Part model, mm, in its own coordinate system. Give positions to 0.01 mm unless a question says otherwise; leave off trailing zeros. Loops run counter-clockwise (first coordinate to the right, second up) from the corner with the lowest first, then second, coordinate; pieces in that order, holes last. Notation, with made-up numbers: M 26,22.25 L 51,22.25 A21 ccw 51,27.25 Z; hole C -35.75,17 d11. An arc over 180 degrees is marked long. Answer in a Markdown table with one row per item.
from build123d import *

# Parameters (mm, degrees)
F1_DEPTH = 3
F2_W     = 55
F2_H     = 3
F3_DEPTH = 60
F5_DEPTH = 3.001
F6_R     = 1.5
F7_DEPTH = 25


with BuildPart() as f1:
    # F0 (on Front) → F1 (new body)
    with BuildSketch(Plane.XZ):
        Polygon((9.642301, -72.468617), (5.525627, -158.370032), (60.462578, -161.002788), (64.579252, -75.101374), (66.01405, -46.877436), (66.01405, -14.442657), (58.229018, -14.069573), (56.766827, -18.181978), (54.847706, -20.834833), (52.745808, -22.111611), (27.019382, -20.834833), (25.082963, -19.47934), (23.824289, -16.671533), (22.565616, -12.120947), (14.142194, -11.443201), (11.49178, -42.476468), align=None)
        Polygon((13.504524, -137.123708), (10.295481, -136.96992), (11.250439, -117.043101), (14.459482, -117.196889), align=None, mode=Mode.SUBTRACT)
        Polygon((59.128299, -119.856104), (58.201853, -139.597923), (54.832633, -139.664747), (55.769612, -119.698487), align=None, mode=Mode.SUBTRACT)
        Polygon((18.496964, -51.870942), (15.419618, -51.640142), (16.890456, -31.622363), (19.998123, -31.855437), align=None, mode=Mode.SUBTRACT)
        Polygon((58.493998, -54.062121), (58.493998, -33.956718), (61.623972, -34.191465), (61.623972, -54.296868), align=None, mode=Mode.SUBTRACT)
    extrude(amount=F1_DEPTH)

    # F2 (on face) → F3 (join)
    with BuildSketch(Plane(origin=(-7.559553, 0, -157.742947), x_dir=(0.998854, 0, -0.047868), z_dir=(-0.047868, 0, -0.998854))):
        with Locations((40.600197, 1.5)):
            Rectangle(F2_W, F2_H)
    extrude(amount=F3_DEPTH)

    # F4 (on face) → F5 (cut, through all)
    with BuildSketch(Plane.XZ.offset(3)):
        Polygon((18.223862, -67.019004), (16.881835, -95.022686), (16.534084, -102.279096), (19.530645, -102.4227), (21.227305, -67.019004), (18.223862, -66.875069), align=None)
        Polygon((53.568468, -68.568897), (51.871808, -103.972594), (54.868369, -104.116199), (55.21612, -96.859789), (56.558147, -68.856107), (56.571911, -68.712832), align=None)
    extrude(amount=-F5_DEPTH, mode=Mode.SUBTRACT)

    # F6 (on face) → F7 (cut)
    with BuildSketch(Plane.XZ.offset(3)):
        with Locations((16.040714, -147.861324)):
            Circle(F6_R)
        with Locations((51.000592, -149.536715)):
            Circle(F6_R)
        with Locations((13.120748, -208.791397)):
            Circle(F6_R)
        with Locations((48.080626, -210.466788)):
            Circle(F6_R)
        Polygon((17.827806, -215.023861), (42.799148, -216.220568), (42.942753, -213.224008), (17.971411, -212.0273), align=None)
    extrude(amount=-F7_DEPTH, mode=Mode.SUBTRACT)


solid = f1.part
(1) Drill centre lines: line 1 along X through (y, z) = (-1.8, -127); line 2 along X through (y, z) = (-1.45, -124); line 3 along Z through (x, y) = (50, -1.4). Where is each one in solid material? Low to high.
Recorded:
| item | result |
|---|---|
| line 1 | x = 7.03 to 10.77, 13.99 to 55.43, 58.79 to 62.09 |
| line 2 | x = 7.17 to 10.92, 14.13 to 55.57, 58.93 to 62.24 |
| line 3 | z = -220.57 to -150.65, -148.42 to -21.98 |
(2) Saw through at C-C (z = -28). Write the cut outline in (x, y).
Recorded:
| item | result |
|---|---|
| outline | M 12.73,-3 L 66.01,-3 L 66.01,0 L 12.73,0 Z |
(3) Saw through at B-B (z = -205.5). Write the cut outline in (x, y).
Recorded:
| item | result |
|---|---|
| outline | M 3.27,-3 L 58.33,-3 L 58.33,0 L 3.27,0 Z |
(4) Saw through at A-A (y = -2.15). Give the number of separate pieces and of enclosed holes in the cut face, plus the area to 3 significant figures.
Recorded:
| item | result |
|---|---|
| separate pieces | 1 |
| enclosed holes | 11 |
| area | 10,500 mm^2 |
(5) Pull direction Y, two halves, no side cores. Call faces 1 (the face through (35, -3, -115)), 2 (the face through (35, 0, -115)): +Y half, -Y half, draft (parallel to the pull), parting line (faces both ways), or undercut.
Recorded:
| item | result |
|---|---|
| face 1 | -Y half |
| face 2 | +Y half |
(6) Pin check, flat tip, straight feed: pin 1 Ø0.9 at (y, z) = (-1.5, -43.5) entering from -X. Stop position of the tip, or through.
Recorded:
| item | result |
|---|---|
| pin 1 | stops at x = 11.4 |
